Part model, mm, in its own coordinate system. A direction names the side the tool comes from. Give positions to 0.01 mm unless a question says otherwise; leave off trailing zeros. Order: outer loops, then holes, each group sorted by start corner. A loop starts at its lowest first (then second) coordinate and runs counter-clockwise, first axis right, second up. Notation, with made-up numbers: M 48,30.5 L 92,30.5 A7 cw 92,38.5 Z; hole C 34.5,54.5 d9. An arc over 180 degrees is marked long. Return JSON: item names as keys, results as strings.
from build123d import *

# Parameters (mm, degrees)
CYLINDER024_R               = 5
CYLINDER024_DEPTH           = 2.5
CYLINDER019_R               = 12
CYLINDER019_DEPTH           = 2.5
CYLINDER027_R               = 8
CYLINDER027_DEPTH           = 12.5
CYLINDER026_R               = 12
CYLINDER026_DEPTH           = 12.5
CYLINDER026_PLACEMENT_ANGLE = 1


with BuildPart() as largeplughole:
    # Cylinder024 → Cylinder024 (new body)
    with BuildSketch(Plane.XY):
        Circle(CYLINDER024_R)
    extrude(amount=CYLINDER024_DEPTH)


with BuildPart() as largeplugbase001:
    # Cylinder019 → Cylinder019 (new body)
    with BuildSketch(Plane.XY):
        Circle(CYLINDER019_R)
    extrude(amount=CYLINDER019_DEPTH)

    # Cut008: cut LargePlugHole
    add(largeplughole.part, mode=Mode.SUBTRACT)


with BuildPart() as largeplugwallhole:
    # Cylinder027 → Cylinder027 (new body)
    with BuildSketch(Plane.XY.offset(2.5)):
        Circle(CYLINDER027_R)
    extrude(amount=CYLINDER027_DEPTH)


with BuildPart() as obj1:
    # Cylinder026 → Cylinder026 (new body)
    with BuildSketch(Plane.XY):
        Circle(CYLINDER026_R)
    extrude(amount=CYLINDER026_DEPTH)


with BuildPart() as obj1_1:
    # Cylinder026 placement: moved
    add(obj1.part.moved(Location((0, 0, 2.5))).rotate(Axis((0, 0, 2.5), (0, 0, 1)), CYLINDER026_PLACEMENT_ANGLE))

    # Cut007: cut LargePlugWallHole
    add(largeplugwallhole.part, mode=Mode.SUBTRACT)

    # Fusion028: union LargePlugBase001
    add(largeplugbase001.part)


with BuildPart() as obj1_2:
    # Fusion028 placement: moved
    add(obj1_1.part.moved(Location((0, -47.75, -2.5))))


solid = obj1_2.part
Q1. Two-plate mould, pull along Y, no slides. Class faces 1 (the flat face through (3, -56, 12.5)), 2 (the cylindrical face through (11.443, -44.136, 4.895)), 3 (the flat face through (-4, -51, 0)): +Y half, -Y half, draft (parallel to the pull), parting line (faces both ways), or undercut.
Established:
{"face 1": "draft", "face 2": "parting line", "face 3": "undercut"}
Q2. Band-saw the part on C-C (x = 3.25). Give the cut face in (y, z), then the cut area to 3 significant figures.
Established:
{"outline": "M -59.3,-2.5 L -51.55,-2.5 L -51.55,0 L -55.06,0 L -55.06,12.5 L -59.3,12.5 Z; M -43.95,-2.5 L -36.2,-2.5 L -36.2,12.5 L -40.44,12.5 L -40.44,0 L -43.95,0 Z", "area": "145 mm²"}
Q3. Probe line 1 along Y through (x, z) = (0, -1.55); line 2 along Y through (x, z) = (0, 7); line 3 along Z through (x, y) = (5.5, -44.25). List the from-to ranges inside material, lowest first.
Established:
{"line 1": "y = -59.75 to -52.75, -42.75 to -35.75", "line 2": "y = -59.75 to -55.75, -39.75 to -35.75", "line 3": "z = -2.5 to 0"}
Q4. 3-axis set-ups, long thin cutter, end or side, ignore diameter. For faces 4 (the cylindrical face through (-1.041, -39.818, 6.162)), 5 (the flat face through (0, -53, -2.5)): which of +Z, -Z, +X, -X, +Y, -Y reach the whole face in a straight line?
Established:
{"face 4": "+Z", "face 5": "-Z, +X, -X, +Y, -Y"}
Q5. Band-saw the part on B-B (z = -1.25). Give the cut face in (x, y).
Established:
{"outline": "C 0,-47.75 d24; hole C 0,-47.75 d10"}
Q6. Band-saw the part on A-A (x = 0). Give the cut face in (y, z).
Established:
{"outline": "M -59.75,-2.5 L -52.75,-2.5 L -52.75,0 L -55.75,0 L -55.75,12.5 L -59.75,12.5 Z; M -42.75,-2.5 L -35.75,-2.5 L -35.75,12.5 L -39.75,12.5 L -39.75,0 L -42.75,0 Z"}
Q7. Band-saw the part on D-D (y = -54). Give the cut face in (x, z), then the cut area to 3 significant figures.
Established:
{"outline": "M -10.24,-2.5 L 10.24,-2.5 L 10.24,12.5 L 4.99,12.5 L 4.99,0 L -4.99,0 L -4.99,12.5 L -10.24,12.5 Z", "area": "182 mm²"}
Q8. Pin check, flat tips, straight feed: pin 1 (9 mm diameter, centred on x = 0, y = -47.75, fed in from -Z); pin 2 (5 mm diameter, centred on x = -4, z = 3.5, fed in from -Y); pin 3 (3 mm diameter, centred on y = -55.5, z = 8, fed in from -X); pin 4 (2 mm diameter, centred on x = -7.5, z = 10.5, fed in from -Y). Stop position of each tip, or through.
Established:
{"pin 1": "passes through", "pin 2": "stops at y = -59.66", "pin 3": "stops at x = -10.24", "pin 4": "stops at y = -57.84"}
